Source: CAD feature listing. Evaluate the final solid. Frame: model axes, mm. Face numbers are marked on the shaded views. A direction names the side the tool comes from. Give positions to 0.01 mm unless a question says otherwise; leave off trailing zeros. Loops run counter-clockwise (first coordinate to the right, second up) from the corner with the lowest first, then second, coordinate; pieces in that order, holes last. Notation, with made-up numbers: (-4, 84) -> (51, 84) arc R22 cw to (51, 113) -> close; hole circle Ø9 at (81, 31.25). An arc over 180 degrees is marked (long way). Return JSON: item names as keys, results as strings. Group by question number.
(1) Pin query (flat end, axial travel): pin 1 (4 mm diameter, centred on y = -57.5, z = -16, fed in from +X); pin 2 (1.5 mm diameter, centred on x = -21.5, y = -37, fed in from +Z); pin 3 (1 mm diameter, centred on x = -18, y = -18, fed in from +Z); pin 4 (24 mm diameter, centred on x = 4, z = -13.5, fed in from +Y). Return the tip coordinate at first contact, or that it passes through.
(2) Cut plane B-B on y = -21. Give the number of separate pieces and of enclosed holes in the cut face, then the cut area to 3 significant figures.
(3) Ray query, line 1 (Y direction, x = 20, z = -35.5); line 2 (Y direction, x = 36.25, z = 0); line 3 (X direction, y = -55.5, z = 0). Return the intervals inside material, ascending. Write a range as from..to.
(4) Cut plane A-A on y = -45. Return loops of the section in (x, z), then the cut area to 3 significant figures.
(5) Access query for the marked faces 4, 5 and 6. Directions: +Z, -Z, +X, -X, +Y, -Y. A direction counts if a zero-diameter tool reaches every point of the face in a straight line with its end or side. Return the directions, or none.
(6) Draft query along Z for the marked faces 1, 2 and 3. Return one class per face: released by +Z, released by -Z, zero draft, split by the parting line, or undercut.
```python
from build123d import *

# Parameters (mm, degrees)
SKETCH_1_R               = 43
EXTRUDE_1_DEPTH          = 70
SKETCH_2_W               = 5
SKETCH_2_H               = 2
SKETCH_2_H_2             = 4
SKETCH_3_R               = 37
CUT_EXTRUDE_1_DEPTH      = 58
EXTRUDE_2_REACH          = 106.757
EXTRUDE_2_END_RADIUS     = 37
SKETCH_4_R               = 15
SKETCH_5_R               = 11
CUT_EXTRUDE_2_DEPTH      = 87
SKETCH_6_R               = 15
CUT_EXTRUDE_3_DEPTH      = 2
SKETCH_7_R               = 1.5
CUT_EXTRUDE_4_DEPTH      = 3.5
PATTERN_CIRCULAR_1_COUNT = 8
CHAMFER_1_SIZE           = 1


with BuildPart() as part:
    # 草图1 → 凸台-拉伸1 (new body)
    with BuildSketch(Plane(origin=(0, 0, 0), x_dir=(1, 0, 0), z_dir=(0, 1, 0))):
        with Locations(Location((0, 0, 0), (0, 0, 270))):
            Circle(SKETCH_1_R)
    extrude(amount=-EXTRUDE_1_DEPTH)

    # 草图2 → 切除-旋转1 (revolve, cut)
    with BuildSketch(Plane.XY, mode=Mode.PRIVATE) as cut_revolve_1_sk:
        with Locations((41.5, -8)):
            Rectangle(SKETCH_2_W, SKETCH_2_H)
        with Locations((41.5, -14)):
            Rectangle(SKETCH_2_W, SKETCH_2_H)
        with Locations((41.5, -21)):
            Rectangle(SKETCH_2_W, SKETCH_2_H_2)
    revolve(cut_revolve_1_sk.sketch.rotate(Axis((0, 0, 0), (0, -1, 0)), 90), axis=Axis((0, 0, 0), (0, -1, 0)), mode=Mode.SUBTRACT)

    # 草图3 → 切除-拉伸1 (cut)
    with BuildSketch(Plane(origin=(0, -70, 0), x_dir=(1, 0, 0), z_dir=(0, 1, 0))):
        with Locations(Location((0, 0, 0), (0, 0, 90))):
            Circle(SKETCH_3_R)
    extrude(amount=CUT_EXTRUDE_1_DEPTH, mode=Mode.SUBTRACT)

    # 凸台-拉伸2: up to this cylinder (the profile starts inside it)
    extrude_2_end = Plane(origin=(0, -40, 0), z_dir=(0, -1, 0)) * Cylinder(EXTRUDE_2_END_RADIUS, 288.514, mode=Mode.PRIVATE)
    # 草图4 → 凸台-拉伸2 (add, up to the surface)
    with BuildSketch(Plane(origin=(22, 0, 0), x_dir=(0, 0, -1), z_dir=(1, 0, 0)), mode=Mode.PRIVATE) as extrude_2_sk1:
        with Locations(Location((0, -40, 0), (0, 0, 180))):
            Circle(SKETCH_4_R)
    extrude_2_tool1 = extrude(extrude_2_sk1.sketch, amount=EXTRUDE_2_REACH, mode=Mode.PRIVATE) & extrude_2_end
    extrude_2 = extrude_2_tool1.solids().sort_by_distance((22, -40, 0))[0]
    add(extrude_2)

    # 镜向1: 凸台-拉伸2 across plane
    add(extrude_2.mirror(Plane(origin=(0, 0, 0), x_dir=(0, 0, 1), z_dir=(1, 0, 0))))

    # 草图5 → 切除-拉伸2 (cut, symmetric)
    with BuildSketch(Plane(origin=(0, 0, 0), x_dir=(0, 0, -1), z_dir=(1, 0, 0))):
        with Locations((0, -40)):
            Circle(SKETCH_5_R)
    extrude(amount=CUT_EXTRUDE_2_DEPTH, both=True, mode=Mode.SUBTRACT)

    # 草图6 → 切除-拉伸3 (cut)
    with BuildSketch(Plane(origin=(0, 0, 0), x_dir=(1, 0, 0), z_dir=(0, 1, 0))):
        with Locations(Location((0, -18, 0), (0, 0, 270))):
            Circle(SKETCH_6_R)
        with Locations(Location((0, 18, 0), (0, 0, 270))):
            Circle(SKETCH_6_R)
    extrude(amount=-CUT_EXTRUDE_3_DEPTH, mode=Mode.SUBTRACT)

    # 草图7 → 切除-拉伸4 (cut)
    with BuildSketch(Plane(origin=(39, 0, 0), x_dir=(0, 0, -1), z_dir=(1, 0, 0))):
        with Locations((0, -21)):
            Circle(SKETCH_7_R)
    cut_extrude_4 = extrude(amount=-CUT_EXTRUDE_4_DEPTH, mode=Mode.SUBTRACT)

    # 阵列(圆周)1: 切除-拉伸4 ×8 about axis
    pattern_circular_1_axis = Axis((0, -73.5, 0), (0, 1, 0))
    for i in range(1, PATTERN_CIRCULAR_1_COUNT):
        add(cut_extrude_4.rotate(pattern_circular_1_axis, i * 360 / PATTERN_CIRCULAR_1_COUNT), mode=Mode.SUBTRACT)

    # 倒角1
    chamfer_1_edges = [part.edges().sort_by_distance(p)[0] for p in [
        (0, 0, -43),
    ]]
    chamfer(chamfer_1_edges, length=CHAMFER_1_SIZE)


solid = part.part
```
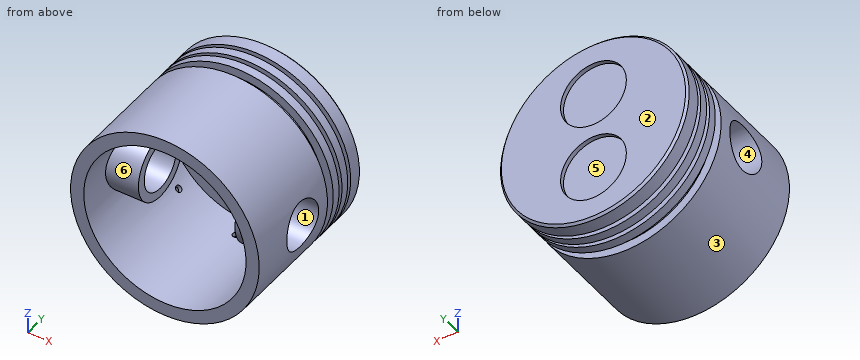
Answers:
{
 "1": {"pin 1": "x = 40.66", "pin 2": "z = 37.66", "pin 3": "z = 39.28", "pin 4": "y = 0"},
 "2": {"separate pieces": "8", "enclosed holes": "0", "area": "430 mm²"},
 "3": {"line 1": "-70..-23, -19..-15, -13..-9, -7..0", "line 2": "-55..-51, -29..-25, -12..0", "line 3": "-43..-37, 37..43"},
 "4": {"outline": "(-41.87, -9.8) arc R43 ccw to (41.87, -9.8) -> (22, -9.8) -> (22, -14.14) -> (34.19, -14.14) arc R37 cw to (-34.19, -14.14) -> (-22, -14.14) -> (-22, -9.8) -> close; (-41.87, 9.8) -> (-22, 9.8) -> (-22, 14.14) -> (-34.19, 14.14) arc R37 cw to (34.19, 14.14) -> (22, 14.14) -> (22, 9.8) -> (41.87, 9.8) arc R43 ccw to start", "area": "1,500 mm²"},
 "5": {"face 4": "+X, -X", "face 5": "+Y", "face 6": "none"},
 "6": {"face 1": "undercut", "face 2": "zero draft", "face 3": "split by the parting line"}
}
